```python
from build123d import *

# Parameters (mm, degrees)
SKETCH1_W                        = 138.42
SKETCH1_H                        = 138.42
SKETCH1_R                        = 2.125
BOSS_EXTRUDE1_DEPTH              = 8
SKETCH2_W                        = 100
SKETCH2_H                        = 100
CUT_EXTRUDE10_DEPTH              = 99.204114985
BOSS_EXTRUDE12_REACH             = 100.204
SKETCH12_W                       = 5
SKETCH12_H                       = 8
BOSS_EXTRUDE12_DIRECTION_2_REACH = 100.204
LPATTERN2_COUNT                  = 6
LPATTERN2_PITCH                  = 23
SKETCH2_3_W                      = 100
SKETCH2_3_H                      = 100
CUT_EXTRUDE13_DEPTH              = 4


with BuildPart() as part:
    # Sketch1 → Boss-Extrude1 (new body)
    with BuildSketch(Plane.XY):
        Rectangle(SKETCH1_W, SKETCH1_H)
        with Locations((-59.285, 59.285)):
            Circle(SKETCH1_R, mode=Mode.SUBTRACT)
        with Locations(Location((59.285, -59.285, 0), (0, 0, 180))):
            Circle(SKETCH1_R, mode=Mode.SUBTRACT)
        with Locations((59.285, 59.285)):
            Circle(SKETCH1_R, mode=Mode.SUBTRACT)
        with Locations(Location((-59.285, -59.285, 0), (0, 0, 180))):
            Circle(SKETCH1_R, mode=Mode.SUBTRACT)
    extrude(amount=BOSS_EXTRUDE1_DEPTH)

    # Sketch2 → Cut-Extrude10 (cut, through all)
    with BuildSketch(Plane.XY.offset(8)):
        Rectangle(SKETCH2_W, SKETCH2_H)
    extrude(amount=-CUT_EXTRUDE10_DEPTH, mode=Mode.SUBTRACT)

    # Sketch12 → Boss-Extrude12 (add, up to next)
    with BuildSketch(Plane(origin=(0, 0, 0), x_dir=(-0.7071067811865477, -0.7071067811865475, 0), z_dir=(0.7071067811865475, -0.7071067811865477, 0)), mode=Mode.PRIVATE) as boss_extrude12_sk1:
        with Locations((-68.210678119, -4)):
            Rectangle(SKETCH12_W, SKETCH12_H)
    boss_extrude12_tool1 = extrude(boss_extrude12_sk1.sketch, amount=BOSS_EXTRUDE12_REACH, mode=Mode.PRIVATE) - part.part
    boss_extrude12 = boss_extrude12_tool1.solids().sort_by_distance((48.232233, 48.232233, 4))[0]
    add(boss_extrude12)

    # Sketch12 → Boss-Extrude12 direction 2 (add, up to next)
    with BuildSketch(Plane(origin=(0, 0, 0), x_dir=(-0.7071067811865477, -0.7071067811865475, 0), z_dir=(0.7071067811865475, -0.7071067811865477, 0)), mode=Mode.PRIVATE) as boss_extrude12_direction_2_sk1:
        with Locations((-68.210678119, -4)):
            Rectangle(SKETCH12_W, SKETCH12_H)
    boss_extrude12_direction_2_tool1 = extrude(boss_extrude12_direction_2_sk1.sketch, amount=-BOSS_EXTRUDE12_DIRECTION_2_REACH, mode=Mode.PRIVATE) - part.part
    boss_extrude12_direction_2 = boss_extrude12_direction_2_tool1.solids().sort_by_distance((48.232233, 48.232233, 4))[0]
    add(boss_extrude12_direction_2)

    # LPattern2: Boss-Extrude12, Boss-Extrude12 direction 2; each copy of Boss-Extrude12, Boss-Extrude12 direction 2 runs up to whatever stops it at its own place
    lpattern2_before = part.part  # the part as the pattern finds it: every copy runs up to it
    lpattern2_boss_extrude12_long = extrude(boss_extrude12_sk1.sketch, amount=BOSS_EXTRUDE12_REACH, mode=Mode.PRIVATE)
    lpattern2_boss_extrude12_tool1 = lpattern2_boss_extrude12_long.moved(Location(Vector(-0.7071067811865477, -0.7071067811865475, 0) * (1 * LPATTERN2_PITCH))) - lpattern2_before
    add(lpattern2_boss_extrude12_tool1.solids().sort_by_distance((31.968777, 31.968777, 4))[0])
    lpattern2_boss_extrude12_tool2 = lpattern2_boss_extrude12_long.moved(Location(Vector(-0.7071067811865477, -0.7071067811865475, 0) * (2 * LPATTERN2_PITCH))) - lpattern2_before
    add(lpattern2_boss_extrude12_tool2.solids().sort_by_distance((15.705321, 15.705321, 4))[0])
    lpattern2_boss_extrude12_tool3 = lpattern2_boss_extrude12_long.moved(Location(Vector(-0.7071067811865477, -0.7071067811865475, 0) * (3 * LPATTERN2_PITCH))) - lpattern2_before
    add(lpattern2_boss_extrude12_tool3.solids().sort_by_distance((-0.558135, -0.558135, 4))[0])
    lpattern2_boss_extrude12_tool4 = lpattern2_boss_extrude12_long.moved(Location(Vector(-0.7071067811865477, -0.7071067811865475, 0) * (4 * LPATTERN2_PITCH))) - lpattern2_before
    add(lpattern2_boss_extrude12_tool4.solids().sort_by_distance((-16.821591, -16.821591, 4))[0])
    lpattern2_boss_extrude12_tool5 = lpattern2_boss_extrude12_long.moved(Location(Vector(-0.7071067811865477, -0.7071067811865475, 0) * (5 * LPATTERN2_PITCH))) - lpattern2_before
    add(lpattern2_boss_extrude12_tool5.solids().sort_by_distance((-33.085047, -33.085047, 4))[0])
    lpattern2_boss_extrude12_direction_2_long = extrude(boss_extrude12_direction_2_sk1.sketch, amount=-BOSS_EXTRUDE12_DIRECTION_2_REACH, mode=Mode.PRIVATE)
    lpattern2_boss_extrude12_direction_2_tool1 = lpattern2_boss_extrude12_direction_2_long.moved(Location(Vector(-0.7071067811865477, -0.7071067811865475, 0) * (1 * LPATTERN2_PITCH))) - lpattern2_before
    add(lpattern2_boss_extrude12_direction_2_tool1.solids().sort_by_distance((31.968777, 31.968777, 4))[0])
    lpattern2_boss_extrude12_direction_2_tool2 = lpattern2_boss_extrude12_direction_2_long.moved(Location(Vector(-0.7071067811865477, -0.7071067811865475, 0) * (2 * LPATTERN2_PITCH))) - lpattern2_before
    add(lpattern2_boss_extrude12_direction_2_tool2.solids().sort_by_distance((15.705321, 15.705321, 4))[0])
    lpattern2_boss_extrude12_direction_2_tool3 = lpattern2_boss_extrude12_direction_2_long.moved(Location(Vector(-0.7071067811865477, -0.7071067811865475, 0) * (3 * LPATTERN2_PITCH))) - lpattern2_before
    add(lpattern2_boss_extrude12_direction_2_tool3.solids().sort_by_distance((-0.558135, -0.558135, 4))[0])
    lpattern2_boss_extrude12_direction_2_tool4 = lpattern2_boss_extrude12_direction_2_long.moved(Location(Vector(-0.7071067811865477, -0.7071067811865475, 0) * (4 * LPATTERN2_PITCH))) - lpattern2_before
    add(lpattern2_boss_extrude12_direction_2_tool4.solids().sort_by_distance((-16.821591, -16.821591, 4))[0])
    lpattern2_boss_extrude12_direction_2_tool5 = lpattern2_boss_extrude12_direction_2_long.moved(Location(Vector(-0.7071067811865477, -0.7071067811865475, 0) * (5 * LPATTERN2_PITCH))) - lpattern2_before
    add(lpattern2_boss_extrude12_direction_2_tool5.solids().sort_by_distance((-33.085047, -33.085047, 4))[0])

    # Sketch2<3> → Cut-Extrude13 (cut)
    with BuildSketch(Plane.XY.offset(8)):
        Rectangle(SKETCH2_3_W, SKETCH2_3_H)
    extrude(amount=-CUT_EXTRUDE13_DEPTH, mode=Mode.SUBTRACT)


solid = part.part
```
Here's how the part is built. I have some questions about the finished solid (model axes, mm). A direction names the side the tool comes from. Give positions to 0.01 mm unless a question says otherwise; leave off trailing zeros. Order: outer loops, then holes, each group sorted by start corner. A loop starts at its lowest first (then second) coordinate and runs counter-clockwise, first axis right, second up. Notation, with made-up numbers: (-31.5, 15) -> (-3.5, 15) arc R20 cw to (-3.5, 44) -> close; hole circle Ø1 at (53.5, 44.25). An arc over 180 degrees is marked (long way). Use CSV: the item, a comma, the result in double quotes. Start each with the question number.
Item 1: Thinking about a two-plate mould opening in Y: for faces 4 (the flat face through (2, 0, 0)), 5 (the flat face through (-1, 69.21, 4)), 6 (the flat face through (-14.565, -15.543, 2.028)), 7 (the flat face through (-1.66, -2.99, 2.03)), which applies, pulls with the +Y half, pulls with the -Y half, needs draft (parallel to the pull), parting line crosses it, or undercut?
Item 2: I'm going to push flat-ended pins straight in: P1, Ø7, axis at x = 59.285, y = -59.285, coming from the -Z side; P2, Ø18.5, axis at x = -25, y = -30.5, coming from the +Z side; P3, Ø3.5, axis at x = 59.285, y = 59.285, coming from the -Z side. Where does each tip first touch, or does it pass through?
Item 3: If I drill on probe 1 along Y at (x, z) = (24.5, 3.5); probe 2 along Y at (x, z) = (-0.5, 7.25); probe 3 along Y at (x, z) = (-58.5, 1.25), over which ranges is the centre line in solid material (lowest first)? Write a range as [from, to].
Item 4: Suppose I cut it at B-B (x = 27). List the corners of the cut face in (y, z) for me.
Item 5: Suppose I cut it at C-C (z = 1.5). Give the number of separate pieces and of enclosed holes in the cut face, and give its area (3 significant figures).
Item 6: Suppose I cut it at A-A (y = -17.5). List the corners of the cut face in (x, z) for me, and give its area (3 significant figures).
Item 7: On a 3-axis mill with a long thin cutter (end or side, diameter ignored), from which of +Z, -Z, +X, -X, +Y, -Y can I reach the whole of each face in a straight line? I mean faces 1 (the flat face through (32, 32, 4)), 2 (the flat face through (1, 51, 8)), 3 (the flat face through (46.514, 46.415, 2.028)). Say none if no direction works.
Answer block:
1,face 4,"needs draft"
1,face 5,"pulls with the +Y half"
1,face 6,"undercut"
1,face 7,"undercut"
2,P1,"stops at z = 0"
2,P2,"stops at z = 4"
2,P3,"passes through"
3,probe 1,"y = [-69.21, -50], [-29.15, -22.08], [3.38, 10.45], [35.9, 42.97], [50, 69.21]"
3,probe 2,"y = [-69.21, -50], [50, 69.21]"
3,probe 3,"y = [-69.21, -61.26], [-57.31, 57.31], [61.26, 69.21]"
4,outline,"(-69.21, 0) -> (-50, 0) -> (-50, 8) -> (-69.21, 8) -> close; (-31.65, 0) -> (-24.58, 0) -> (-24.58, 4) -> (-31.65, 4) -> close; (0.88, 0) -> (7.95, 0) -> (7.95, 4) -> (0.88, 4) -> close; (33.4, 0) -> (40.47, 0) -> (40.47, 4) -> (33.4, 4) -> close; (50, 0) -> (69.21, 0) -> (69.21, 8) -> (50, 8) -> close"
5,separate pieces,"1"
5,enclosed holes,"10"
5,area,"11,300 mm^2"
6,outline,"(-69.21, 0) -> (-45.13, 0) -> (-45.13, 4) -> (-50, 4) -> (-50, 8) -> (-69.21, 8) -> close; (-19.68, 0) -> (-12.61, 0) -> (-12.61, 4) -> (-19.68, 4) -> close; (12.85, 0) -> (19.92, 0) -> (19.92, 4) -> (12.85, 4) -> close; (45.38, 0) -> (69.21, 0) -> (69.21, 8) -> (50, 8) -> (50, 4) -> (45.38, 4) -> close"
6,area,"402 mm^2"
7,face 1,"+Z"
7,face 2,"+Z, +X, -X, +Y, -Y"
7,face 3,"+Z, -Z"
